from build123d import *

# Parameters (mm, degrees)
BOSS_EXTRUDE1_DEPTH = 60
FILLET1_R           = 10
FILLET2_R           = 10
SKETCH2_R           = 10
CUT_EXTRUDE1_DEPTH  = 60


with BuildPart() as part:
    # Sketch1 → Boss-Extrude1 (new body)
    with BuildSketch(Plane.XY):
        Polygon((0, 0), (0, 100), (100, 100), (100, 97), (3, 97), (3, 0), align=None)
    extrude(amount=BOSS_EXTRUDE1_DEPTH)

    # Fillet1
    fillet1_edges = [part.edges().sort_by_distance(p)[0] for p in [
        (100, 98.5, 60),
        (100, 98.5, 0),
    ]]
    fillet(fillet1_edges, radius=FILLET1_R)

    # Fillet2
    fillet2_edges = [part.edges().sort_by_distance(p)[0] for p in [
        (1.5, 0, 60),
        (1.5, 0, 0),
    ]]
    fillet(fillet2_edges, radius=FILLET2_R)

    # Sketch2 → Cut-Extrude1 (cut)
    with BuildSketch(Plane(origin=(3, 0, 0), x_dir=(0, 0, -1), z_dir=(1, 0, 0))):
        with Locations((-30, 40)):
            Circle(SKETCH2_R)
        with Locations((-30, 80)):
            Circle(SKETCH2_R)
    extrude(amount=-CUT_EXTRUDE1_DEPTH, mode=Mode.SUBTRACT)


solid = part.part
Design review of the part built by this model. Coordinates are the model's own, in mm. A direction names the side the tool comes from. Coordinates: 2 decimals unless noted, no trailing zeros. Order: outer loops, then holes, each group sorted by start corner. A loop starts at its lowest first (then second) coordinate and runs counter-clockwise, first axis right, second up.
Item 1: Take a section at C-C, the plane x = 75. Write out the cut boundary in (y, z).
Item 2: Take a section at D-D, the plane z = 6.5. Write out the cut boundary in (x, y).
Item 3: For faces 1 (the flat face through (3, 49, 36)), 2 (the flat face through (2, 75, 60)), list the 3-axis set-ups (+Z, -Z, +X, -X, +Y, -Y) from which the entire face can be reached by the end or side of a thin tool; tool diameter is ignored.
Item 4: For line 1 (Y direction, x = 2.45, z = 30); line 2 (Y direction, x = 25, z = 39.5); line 3 (X direction, y = 73.5, z = 11.5), list the stretches that pass through material, from the lowest coordinate up.
Item 5: The part is to be moulded in two halves that separate along Y. For faces 3 (the cylindrical face through (1.521, 89.915, 31.302)), 4 (the flat face through (0, 49, 36)), 5 (the flat face through (49, 100, 30)), 6 (the cylindrical face through (1.48, 3.01, 2.85)), say which applies: pulls with the +Y half, pulls with the -Y half, needs draft (parallel to the pull), parting line crosses it, or undercut.
Item 6: Take a section at B-B, the plane y = 88. Write out the cut boundary in (x, z), then the cut area to 3 significant figures.
Item 7: Take a section at A-A, the plane z = 30. Write out the cut boundary in (x, y), then the cut area to 3 significant figures.
Item 8: For pin 1 Ø4 at (x, z) = (73.5, 24) entering from -Y; pin 2 Ø1.5 at (y, z) = (50.5, 49.5) entering from -X; pin 3 Ø1 at (y, z) = (87, 23) entering from +X, all flat-tipped, find the tip position at first contact; note any pin that passes through.
The answers:
1. outline: (97, 0) - (100, 0) - (100, 60) - (97, 60) - close
2. outline: (0, 0.63) - (3, 0.63) - (3, 97) - (99.37, 97) - (99.37, 100) - (0, 100) - close
3. face 1: +Z, -Z, +X, -Y
3. face 2: +Z, +X, -X, +Y, -Y
4. line 1: y = 0 to 30, 50 to 70, 90 to 100
4. line 2: y = 97 to 100
4. line 3: x = 0 to 3
5. face 3: undercut
5. face 4: needs draft
5. face 5: pulls with the +Y half
5. face 6: pulls with the -Y half
6. outline: (0, 0) - (3, 0) - (3, 24) - (0, 24) - close; (0, 36) - (3, 36) - (3, 60) - (0, 60) - close
6. area: 144 mm2
7. outline: (0, 0) - (3, 0) - (3, 30) - (0, 30) - close; (0, 50) - (3, 50) - (3, 70) - (0, 70) - close; (0, 90) - (3, 90) - (3, 97) - (100, 97) - (100, 100) - (0, 100) - close
7. area: 471 mm2
8. pin 1: stops at y = 97
8. pin 2: stops at x = 0
8. pin 3: stops at x = 3
